The model under review builds one solid part; all positions refer to its coordinate system, in mm. A direction names the side the tool comes from. Coordinates: 2 decimals unless noted, no trailing zeros. Write each question's results on one line, items separated by ' | '.
from build123d import *

# Parameters (mm, degrees)
SKETCH1_W               = 37.5
SKETCH1_H               = 50
BOSS_EXTRUDE1_DEPTH     = 55
SKETCH3_R               = 15
BOSS_EXTRUDE2_DEPTH     = 7
SHELL1_T                = -3.5
SKETCH4_R               = 5.121522354
CUT_EXTRUDE1_DEPTH      = 7
CUT_EXTRUDE2_DEPTH      = 72.107313267
CUT_EXTRUDE2_DEPTH_BACK = 72.107313267
SKETCH5_W               = 46
SKETCH5_H               = 25
TAP_DRILL_FOR_M2_TAP1_D = 2
CUT_EXTRUDE4_DEPTH      = 1.5
FILLET1_R               = 1
FILLET2_R               = 0.5
SKETCH11_R              = 11.5
CUT_EXTRUDE5_DEPTH      = 1.5
F_1_0MM_DOWEL_HOLE1_D   = 2


with BuildPart() as part:
    # Sketch1 → Boss-Extrude1 (new body)
    with BuildSketch(Plane.XY):
        Rectangle(SKETCH1_W, SKETCH1_H)
    extrude(amount=BOSS_EXTRUDE1_DEPTH)

    # Sketch3 → Boss-Extrude2 (add)
    with BuildSketch(Plane(origin=(0, 0, 0), x_dir=(-1, 0, 0), z_dir=(0, 0, -1))):
        Circle(SKETCH3_R)
    extrude(amount=BOSS_EXTRUDE2_DEPTH)

    # Shell1
    shell1_openings = [part.faces().sort_by_distance(p)[0] for p in [
        (0, 0, 55),
        (0, 25, 27.5),
    ]]
    offset(amount=SHELL1_T, openings=shell1_openings, kind=Kind.INTERSECTION)

    # Sketch4 → Cut-Extrude1 (cut)
    with BuildSketch(Plane.XY.offset(-3.5)):
        Circle(SKETCH4_R)
    extrude(amount=-CUT_EXTRUDE1_DEPTH, mode=Mode.SUBTRACT)

    # Sketch5 → Cut-Extrude2 (cut, two sides: drawn at the far end of the back side and taken through both)
    with BuildSketch(Plane.ZY.offset(18.75).offset(-CUT_EXTRUDE2_DEPTH_BACK)):
        with Locations((32, 0)):
            Rectangle(SKETCH5_W, SKETCH5_H)
    extrude(amount=CUT_EXTRUDE2_DEPTH + CUT_EXTRUDE2_DEPTH_BACK, mode=Mode.SUBTRACT)

    # Tap Drill for M2 Tap1 (through all)
    with Locations(Plane(origin=(18.75, 15, 46.6), x_dir=(0, 1, 0), z_dir=(1, 0, 0))):
        with Locations((0, 0), (0, -17), (-30, 0), (-30, -17), (-30, -34), (-23.5, -40.3), (-6.5, -40.3), (0, -34)):
            Hole(TAP_DRILL_FOR_M2_TAP1_D / 2)

    # Sketch10 → Cut-Extrude4 (cut)
    with BuildSketch(Plane(origin=(18.75, 0, 0), x_dir=(0, 0, -1), z_dir=(1, 0, 0))):
        with BuildLine():
            Line((-55, -18.25), (-8.5, -18.25))
            ThreePointArc((-8.5, -18.25), (-4.964466094, -16.785533906), (-3.5, -13.25))
            Line((-3.5, -13.25), (-3.5, 13.25))
            ThreePointArc((-3.5, 13.25), (-4.964466094, 16.785533906), (-8.5, 18.25))
            Line((-8.5, 18.25), (-55, 18.25))
            Line((-55, 18.25), (-55, -18.25))
        make_face()
    cut_extrude4 = extrude(amount=-CUT_EXTRUDE4_DEPTH, mode=Mode.SUBTRACT)

    # Mirror1: Cut-Extrude4 across plane
    add(cut_extrude4.mirror(Plane(origin=(0, 0, 0), x_dir=(0, 0, 1), z_dir=(1, 0, 0))), mode=Mode.SUBTRACT)

    # Fillet1
    fillet1_edges = [part.edges().sort_by_distance(p)[0] for p in [
        (15, 0, 0),
        (15.25, -21.5, 29.25),
        (15.25, 25, 29.25),
        (-15.25, 25, 29.25),
        (-15.25, -21.5, 29.25),
        (0, -25, 0),
        (-18.75, 0, 0),
        (0, 25, 0),
        (18.75, 0, 0),
        (18.75, -25, 27.5),
        (-18.75, -25, 27.5),
        (-18.75, 25, 27.5),
        (18.75, 25, 27.5),
    ]]
    fillet(fillet1_edges, radius=FILLET1_R)

    # Fillet2
    fillet2_edges = [part.edges().sort_by_distance(p)[0] for p in [
        (18.75, -18.25, 31.75),
        (18.75, -16.785533906, 4.964466094),
        (18.75, 0, 3.5),
        (18.75, 16.785533906, 4.964466094),
        (18.75, 18.25, 31.75),
        (17.25, 18.25, 31.75),
        (17.25, 16.785533906, 4.964466094),
        (17.25, 0, 3.5),
        (17.25, -16.785533906, 4.964466094),
        (17.25, -18.25, 31.75),
        (-17.25, -18.25, 31.75),
        (-17.25, -16.785533906, 4.964466094),
        (-17.25, 0, 3.5),
        (-17.25, 16.785533906, 4.964466094),
        (-17.25, 18.25, 31.75),
        (-18.75, -18.25, 31.75),
        (-18.75, -16.785533906, 4.964466094),
        (-18.75, 0, 3.5),
        (-18.75, 16.785533906, 4.964466094),
        (-18.75, 18.25, 31.75),
    ]]
    fillet(fillet2_edges, radius=FILLET2_R)

    # Sketch11 → Cut-Extrude5 (cut)
    with BuildSketch(Plane.XY.offset(-3.5)):
        Circle(SKETCH11_R)
    extrude(amount=-CUT_EXTRUDE5_DEPTH, mode=Mode.SUBTRACT)

    # Ø1.0mm Dowel Hole1 (through all)
    with Locations(Plane(origin=(5.656854249, 5.656854249, -5), x_dir=(1, 0, 0), z_dir=(0, 0, 1))):
        with Locations((0, 0), (-5.656854249, 2.343145751), (2.343145751, -5.656854249), (0, -11.313708498), (-5.656854249, -13.656854249), (-11.313708498, -11.313708498), (-13.656854249, -5.656854249), (-11.313708498, 0)):
            Hole(F_1_0MM_DOWEL_HOLE1_D / 2)


solid = part.part
1) To check wall thickness, follow line 1 along X through (y, z) = (19, 41); line 2 along Y through (x, z) = (-16, 29); line 3 along Z through (x, y) = (-2, 11). State the ranges of each line that lie inside material, in increasing order.
Solutions:
line 1: -18.75 to -15.25, 15.25 to 18.75 | line 2: -25 to -15.8, -14.2 to -12.5, 12.5 to 14.2, 15.8 to 24.97 | line 3: -7 to -5
2) Take a section at A-A on x = 0. Count the separate pieces of the cut face and the enclosed holes in it, plus the area to 3 significant figures.
Solutions:
separate pieces: 4 | enclosed holes: 0 | area: 341 mm2
3) For faces 4 (the flat face through (-16, 12.5, 32)), 5 (the flat face through (-17.25, 13, 28)), 6 (the flat face through (5, -2, -5)), list the 3-axis set-ups (+Z, -Z, +X, -X, +Y, -Y) from which the entire face can be reached by the end or side of a thin tool; tool diameter is ignored.
Solutions:
face 4: +Z, +X, -X | face 5: +Z, -X | face 6: +Z
4) For pin 1 (0.6 mm diameter, centred on x = 18, y = 4.5, fed in from +Z); pin 2 (10 mm diameter, centred on x = -6, z = 24, fed in from +Y); pin 3 (6 mm diameter, centred on x = 0, y = 0, fed in from +Z); pin 4 (6 mm diameter, centred on y = -3, z = 7, fed in from +X), all flat-tipped, find the tip position at first contact; note any pin that passes through.
Solutions:
pin 1: z = 3.5 | pin 2: y = -21.5 | pin 3: through | pin 4: x = 17.25
5) The part is to be moulded in two halves that separate along Y. For faces 1 (the flat face through (16, 0, 9)), 2 (the flat face through (17, 25, 20)), 3 (the flat face through (15.25, 16, 29)), say which applies: pulls with the +Y half, pulls with the -Y half, needs draft (parallel to the pull), parting line crosses it, or undercut.
Solutions:
face 1: undercut | face 2: pulls with the +Y half | face 3: needs draft
